Source: CAD feature listing. Evaluate the final solid. Frame: model axes, mm. A direction names the side the tool comes from. Give positions to 0.01 mm unless a question says otherwise; leave off trailing zeros. Loops run counter-clockwise (first coordinate to the right, second up) from the corner with the lowest first, then second, coordinate; pieces in that order, holes last.
Autodesk Inventor part; units mm, degrees
ref_plane "YZ Plane" through (0, 0, 0) normal (1, 0, 0) x (0, 1, 0)
ref_plane "XZ Plane" through (0, 0, 0) normal (0, 1, 0) x (-1, 0, 0)
ref_plane "XY Plane" through (0, 0, 0) normal (0, 0, 1) x (1, 0, 0)
sketch "Sketch1" plane through (0, 0, 0) normal (0, 0, 1) x (1, 0, 0)
  circle A0 centre (0, 0) radius 10.7
  circle A1 centre (8, 0) radius 1.5
  circle A2 centre (0, 8) radius 1.5
  circle A3 centre (0, -8) radius 1.5
  circle A4 centre (0, 0) radius 2
  circle A5 centre (-8, 0) radius 1.5
extrude "Extrusion1" add sketch "Sketch1" along normal blind 2
sketch "Sketch2" plane through (0, 0, 2) normal (0, 0, 1) x (1, 0, 0)
  circle A0 centre (0, 0) radius 2
  circle A1 centre (0, 0) radius 5
  dimension "d2" = 10
extrude "Extrusion2" add sketch "Sketch2" along normal blind 10
properties part number "AcopleBrida4" material "Acero"
1) Ray query, probe 1 along Y at (x, z) = (0, 0.7); probe 2 along Y at (x, z) = (0, 7.75); probe 3 along Z at (x, y) = (6.5, 5.75). Return the intervals inside material, ascending.
Checks:
probe 1: y = -10.7 to -9.5, -6.5 to -2, 2 to 6.5, 9.5 to 10.7
probe 2: y = -5 to -2, 2 to 5
probe 3: z = 0 to 2
2) Contact query for flat-ended pins moving along their axis: P1, Ø3.5, axis at x = 0, y = -8, coming from the +Z side; P2, Ø2.5, axis at x = -8, y = 0, coming from the +Z side; P3, Ø2, axis at x = -1.5, z = 9, coming from the -Y side; P4, Ø5, axis at y = 4, z = 1.5, coming from the -X side. Output: stop coordinate, or through.
Checks:
P1: stops at z = 2
P2: passes through
P3: stops at y = -4.97
P4: stops at x = -10.59
3) Cut plane A-A (x = 0). Return loops of the section in (y, z), and give its area (3 significant figures).
Checks:
outline: (-10.7, 0) - (-9.5, 0) - (-9.5, 2) - (-10.7, 2) - close; (-6.5, 0) - (-2, 0) - (-2, 12) - (-5, 12) - (-5, 2) - (-6.5, 2) - close; (2, 0) - (6.5, 0) - (6.5, 2) - (5, 2) - (5, 12) - (2, 12) - close; (9.5, 0) - (10.7, 0) - (10.7, 2) - (9.5, 2) - close
area: 82.8 mm2
4) Cut plane D-D (x = 8). Return loops of the section in (y, z), and give its area (3 significant figures).
Checks:
outline: (-7.11, 0) - (-1.5, 0) - (-1.5, 2) - (-7.11, 2) - close; (1.5, 0) - (7.11, 0) - (7.11, 2) - (1.5, 2) - close
area: 22.4 mm2
5) Reachability of faces 1 (the cylindrical face through (-0.325, -6.536, 0.986)), 2 (the flat face through (2, -5, 2)) from +Z, -Z, +X, -X, +Y, -Y: full face, straight path, thin tool, end or side. Return the list, or none.
Checks:
face 1: +Z, -Z
face 2: +Z
6) Pull-direction query (Y, two-part tool) for faces 3 (the cylindrical face through (-0.325, 9.464, 0.986)), 4 (the flat face through (-0.1, -2.2, 0)), 5 (the cylindrical face through (-1.08, 4.88, 6.93)); classes: released by +Y, released by -Y, zero draft, split by the parting line, or undercut.
Checks:
face 3: undercut
face 4: zero draft
face 5: split by the parting line
7) Cut plane C-C (z = 1). Return loops of the section in (x, y), and give its area (3 significant figures).
Checks:
outline: circle Ø21.4 at (0, 0); hole circle Ø3 at (-8, 0); hole circle Ø4 at (0, 0); hole circle Ø3 at (0, -8); hole circle Ø3 at (0, 8); hole circle Ø3 at (8, 0)
area: 319 mm2
